from build123d import *

# Parameters (mm, degrees)
FILLET1_R = 0.4


with BuildPart() as part:
    # Sketch1 → Revolve1 (revolve)
    with BuildSketch(Plane(origin=(0, 0, 0), x_dir=(0, 0, -1), z_dir=(1, 0, 0))):
        Polygon((4, 8), (4, 0), (8, 0), (8, 2), (6, 2), (6, 8), align=None)
    revolve(axis=Axis((0, 0, 0), (0, 1, 0)))

    # Fillet1
    fillet1_edges = [part.edges().sort_by_distance(p)[0] for p in [
        (0, 2, 6),
    ]]
    fillet(fillet1_edges, radius=FILLET1_R)


solid = part.part
Geometry: final body of the model. Coordinates: model frame, mm. A direction names the side the tool comes from. Coordinates: 2 decimals unless noted, no trailing zeros. Order: outer loops, then holes, each group sorted by start corner. A loop starts at its lowest first (then second) coordinate and runs counter-clockwise, first axis right, second up.
(1) Material intervals for probe 1 along Z at (x, y) = (0, 4); probe 2 along Y at (x, z) = (5, -6), sorted ascending.
(2) Section query B-B (z = 0). Return the cut outline in (x, y), plus the area to 3 significant figures.
(3) Draft query along X for faces 1 (the face through (2, 0, -4)), 2 (the face through (3.905, 3.944, 0.867)), 3 (the face through (7.81, 1.01, 1.73)). Return one class per face: pulls with the +X half, pulls with the -X half, needs draft (parallel to the pull), parting line crosses it, or undercut.
(4) Section query A-A (x = 0). Return the cut outline in (y, z).
(5) Access query for faces 4 (the face through (3.92, 8, 1.42)), 5 (the face through (-7, 2, 0)). Directions: +Z, -Z, +X, -X, +Y, -Y. A direction counts if a zero-diameter tool reaches every point of the face in a straight line with its end or side. Return the directions, or none.
(6) Section query C-C (y = 3). Return the cut outline in (x, z), plus the area to 3 significant figures.
(7) First-contact query: pin 1 (1 mm diameter, centred on x = -2.5, y = 1.5, fed in from -Z); pin 2 (4 mm diameter, centred on y = 5.5, z = 3.5, fed in from -X); pin 3 (2 mm diameter, centred on x = 6.5, y = 2.5, fed in from +Z); pin 4 (5 mm diameter, centred on x = 0, z = 0, fed in from -Y). Flat tips, straight axial feed; report the tip coordinate or a pass-through.
Solution:
1. probe 1: z = -6 to -4, 4 to 6
1. probe 2: y = 0 to 2
2. outline: (-8, 0) - (-4, 0) - (-4, 8) - (-6, 8) - (-6, 2.4) arc R0.4 cw to (-6.4, 2) - (-8, 2) - close; (4, 0) - (8, 0) - (8, 2) - (6.4, 2) arc R0.4 cw to (6, 2.4) - (6, 8) - (4, 8) - close
2. area: 40.1 mm2
3. face 1: needs draft
3. face 2: undercut
3. face 3: parting line crosses it
4. outline: (0, -8) - (2, -8) - (2, -6.4) arc R0.4 cw to (2.4, -6) - (8, -6) - (8, -4) - (0, -4) - close; (0, 4) - (8, 4) - (8, 6) - (2.4, 6) arc R0.4 cw to (2, 6.4) - (2, 8) - (0, 8) - close
5. face 4: +Z, -Z, +X, -X, +Y
5. face 5: +Y
6. outline: circle Ø12 at (0, 0); hole circle Ø8 at (0, 0)
6. area: 62.8 mm2
7. pin 1: stops at z = -7.75
7. pin 2: stops at x = -5.81
7. pin 3: stops at z = 5.68
7. pin 4: passes through
